```python
from build123d import *

# Parameters (mm, degrees)
SKETCH_1_W          = 58
SKETCH_1_H          = 58
SKETCH_1_R          = 28
EXTRUDE_1_DEPTH     = 30
SKETCH_2_R          = 5
CUT_EXTRUDE_1_DEPTH = 51.813384064


with BuildPart() as part:
    # 草图1 → 凸台-拉伸1 (new body)
    with BuildSketch(Plane.XY):
        Rectangle(SKETCH_1_W, SKETCH_1_H)
        Circle(SKETCH_1_R, mode=Mode.SUBTRACT)
    extrude(amount=EXTRUDE_1_DEPTH)

    # 草图2 → 切除-拉伸1 (cut, through all)
    with BuildSketch(Plane.XY.offset(30)):
        with Locations((22.9, 22.9)):
            Circle(SKETCH_2_R)
        with Locations((22.9, -22.9)):
            Circle(SKETCH_2_R)
        with Locations((-22.9, -22.9)):
            Circle(SKETCH_2_R)
        with Locations((-22.9, 22.9)):
            Circle(SKETCH_2_R)
    extrude(amount=-CUT_EXTRUDE_1_DEPTH, mode=Mode.SUBTRACT)


solid = part.part
```
Here's how the part is built. I have some questions about the finished solid (model axes, mm). A direction names the side the tool comes from. Round coordinates to 2 decimals unless told otherwise and drop trailing zeros. Order: outer loops, then holes, each group sorted by start corner. A loop starts at its lowest first (then second) coordinate and runs counter-clockwise, first axis right, second up. Notation, with made-up numbers: M 67.25,61 L 104.25,61 A19 ccw 104.25,92 Z; hole C 15.25,48 d8. An arc over 180 degrees is marked long. Answer in a Markdown table with one row per item.
Item 1: Imagine slicing it at C-C, the plane z = 16.5. Write out the boundary of the cut face in (x, y).
A:
| item | result |
|---|---|
| outline | M -29,-29 L 29,-29 L 29,29 L -29,29 Z; hole M -21.31,-18.16 A5 ccw long -18.16,-21.31 A28 ccw 18.16,-21.31 A5 ccw long 21.31,-18.16 A28 ccw 21.31,18.16 A5 ccw long 18.16,21.31 A28 ccw -18.16,21.31 A5 ccw long -21.31,18.16 A28 ccw Z |
Item 2: Imagine slicing it at A-A, the plane y = -0.5. Write out the boundary of the cut face in (x, z).
A:
| item | result |
|---|---|
| outline | M -29,0 L -28,0 L -28,30 L -29,30 Z; M 28,0 L 29,0 L 29,30 L 28,30 Z |
Item 3: Thinking about a two-plate mould opening in X: for faces 3 (the face through (-29, 0, 15)), 4 (the face through (0, -29, 15)), 5 (the face through (29, 0, 15)), 6 (the face through (28, 0, 15)), which applies, +X half, -X half, draft (parallel to the pull), parting line (faces both ways), or undercut?
A:
| item | result |
|---|---|
| face 3 | -X half |
| face 4 | draft |
| face 5 | +X half |
| face 6 | undercut |
Item 4: If I drill on L1, parallel to Y at x = -24, z = 6; L2, parallel to Y at x = 22.9, z = 9, over which ranges is the centre line in solid material (lowest first)? Write a range as from..to.
A:
| item | result |
|---|---|
| L1 | y = -29..-27.78, -18.02..-14.42, 14.42..18.02, 27.78..29 |
| L2 | y = -29..-27.9, -17.9..-16.11, 16.11..17.9, 27.9..29 |
Item 5: Imagine slicing it at B-B, the plane x = 22.9. Write out the boundary of the cut face in (y, z).
A:
| item | result |
|---|---|
| outline | M -29,0 L -27.9,0 L -27.9,30 L -29,30 Z; M -17.9,0 L -16.11,0 L -16.11,30 L -17.9,30 Z; M 16.11,0 L 17.9,0 L 17.9,30 L 16.11,30 Z; M 27.9,0 L 29,0 L 29,30 L 27.9,30 Z |
Item 6: For faces 1 (the face through (0, 29, 15)), 2 (the face through (0, 28, 15)), which set-ups out of +Z, -Z, +X, -X, +Y, -Y let a thin tool reach every point of the face, with its end or its side?
A:
| item | result |
|---|---|
| face 1 | +Z, -Z, +X, -X, +Y |
| face 2 | +Z, -Z |
